Part model, mm, in its own coordinate system. A direction names the side the tool comes from. Round coordinates to 2 decimals unless told otherwise and drop trailing zeros. Write each loop counter-clockwise with the first axis right and the second up, starting at its lowest first coordinate (ties: lowest second). Pieces come first, ordered by that corner, then holes.
1) Flat gauge pin, fed straight in: pin 1 (3 mm diameter, centred on x = 6.5, y = 112.5, fed in from -Z). Where does the tip first touch, or does it go through?
2) Saw through at B-B on z = 52.5. Write the cut outline in (x, y), and give its area (3 significant figures).
3) Saw through at A-A on x = 13. Write the cut outline in (y, z), and give its area (3 significant figures).
4) Saw through at C-C on y = 115. Write the cut outline in (x, z), and give its area (3 significant figures).
5) Drill centre lines: L1, parallel to Y at x = 4.5, z = 15.5; L2, parallel to Z at x = 9.75, y = 114.5. Where is each one in solid material? Low to high.
6) Which spindle directions (+Z, -Z, +X, -X, +Y, -Y) get a long thin tool onto all of the face, cutting with end or side? Do faces 1 (the flat face through (9, 116, 27)), 2 (the flat face through (9, 124, 29)). Say none if no direction does.
```python
from build123d import *

# Parameters (mm, degrees)
BOX018_W                  = 12
BOX018_H                  = 8
BOX018_DEPTH              = 55
BOX017_W                  = 12
BOX017_H                  = 14
BOX017_DEPTH              = 3
FUSION010_PLACEMENT_ANGLE = 180


with BuildPart() as obj1:
    # Box018 → Box018 (new body)
    with BuildSketch(Plane(origin=(47, 17, 0), x_dir=(1, 0, 0), z_dir=(0, 0, 1))):
        with Locations((6, 4)):
            Rectangle(BOX018_W, BOX018_H)
    extrude(amount=BOX018_DEPTH)


with BuildPart() as l3:
    # Box017 → Box017 (new body)
    with BuildSketch(Plane(origin=(47, 17, 55), x_dir=(1, 0, 0), z_dir=(0, 0, 1))):
        with Locations((6, 7)):
            Rectangle(BOX017_W, BOX017_H)
    extrude(amount=BOX017_DEPTH)

    # Fusion010: union obj1
    add(obj1.part)


with BuildPart() as l3_1:
    # Fusion010 placement: moved
    add(l3.part.moved(Location((62, 141, 0))).rotate(Axis((62, 141, 0), (0, 0, 1)), FUSION010_PLACEMENT_ANGLE))


solid = l3_1.part
```
Completed:
1. pin 1: stops at z = 55
2. outline: (3, 116) - (15, 116) - (15, 124) - (3, 124) - close
2. area: 96.0 mm2
3. outline: (110, 55) - (116, 55) - (116, 0) - (124, 0) - (124, 58) - (110, 58) - close
3. area: 482 mm2
4. outline: (3, 55) - (15, 55) - (15, 58) - (3, 58) - close
4. area: 36.0 mm2
5. L1: y = 116 to 124
5. L2: z = 55 to 58
6. face 1: -Z, +X, -X, -Y
6. face 2: +Z, -Z, +X, -X, +Y
